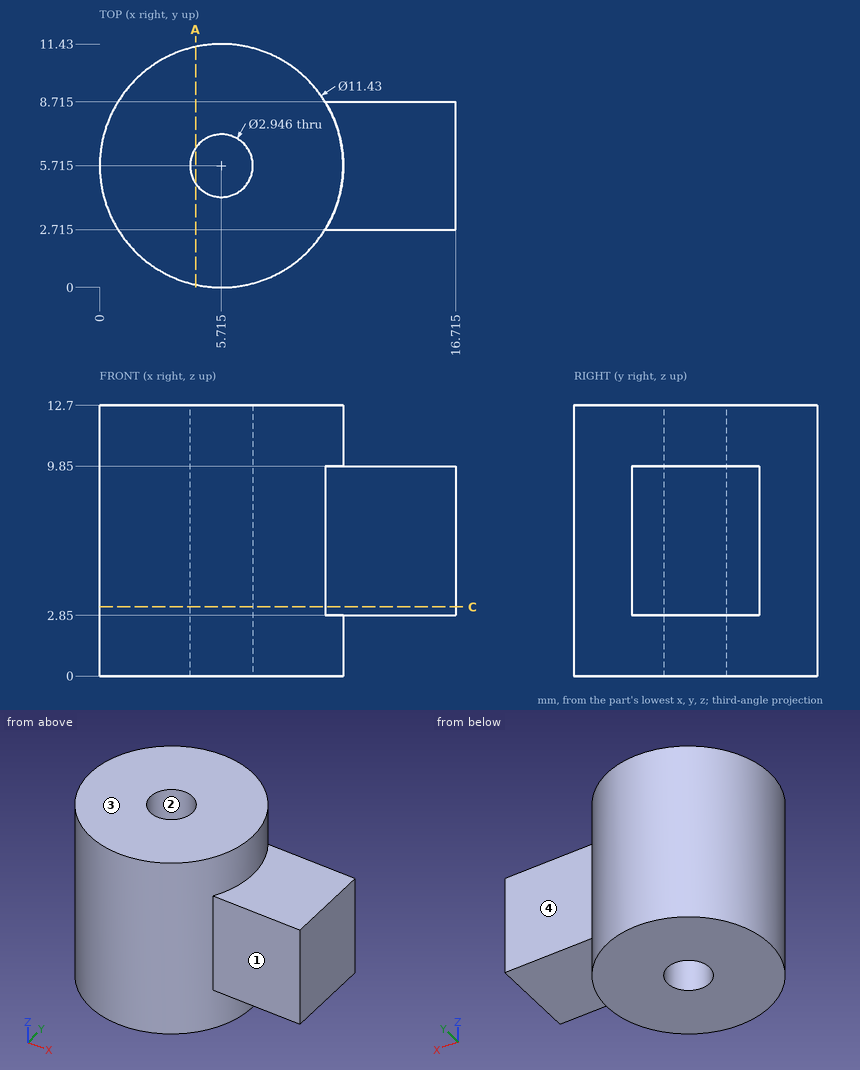
Study the drawing (mm; zero at the part's minimum x, y, z) and answer. Coordinates: 2 decimals unless noted, no trailing zeros. Write each loop counter-clockwise with the first axis right and the second up, starting at its lowest first coordinate (ties: lowest second). Pieces come first, ordered by that corner, then holes.
Q1. Section C-C, the plane z = 3.25 is taken. Write down the section's boundary in (x, y) (1 decimal), then the cut area to 3 significant figures.
Returned:
outline: (10.6, 2.7) - (16.7, 2.7) - (16.7, 8.7) - (10.6, 8.7) arc R5.7 ccw (long way) to start; hole circle Ø2.9 at (5.7, 5.7)
area: 129 mm2
Q2. The mould has two halves that part along Y. Classify the marked faces 1, 2, 3 and 4: released by +Y, released by -Y, zero draft, split by the parting line, or undercut.
Returned:
face 1: released by -Y
face 2: undercut
face 3: zero draft
face 4: released by +Y
Q3. Given P1, Ø3, axis at x = 13.5, z = 5.5, coming from the -Y side (3 decimals); P2, Ø2.5, axis at x = 5.715, y = 5.715, coming from the -Z side; P3, Ø5, axis at y = 3, z = 2, coming from the -X side; P4, Ø2, axis at y = 1.5, z = 2.5, coming from the -X side, each flat-ended and moving along its own axis, determine where each tip first touches the part or whether it passes through.
Returned:
P1: stops at y = 2.715
P2: passes through
P3: stops at x = 0
P4: stops at x = 0.99
Q4. Find the intervals of material crossed by line 1 along Y through (x, z) = (5.75, 8.25); line 2 along Y through (x, z) = (13.25, 9.75) (1 decimal), in increasing order.
Returned:
line 1: y = 0 to 4.24, 7.19 to 11.43
line 2: y = 2.7 to 8.7
Q5. Section A-A, the plane x = 4.5 is taken. Write down the section's boundary in (y, z).
Returned:
outline: (0.13, 0) - (4.88, 0) - (4.88, 12.7) - (0.13, 12.7) - close; (6.55, 0) - (11.3, 0) - (11.3, 12.7) - (6.55, 12.7) - close
